Check sheet for the modelled part. Datum: model origin and axes. Units: mm. Face numbers are marked on the shaded views. A direction names the side the tool comes from. Round coordinates to 2 decimals unless told otherwise and drop trailing zeros. Write each loop counter-clockwise with the first axis right and the second up, starting at its lowest first coordinate (ties: lowest second). Pieces come first, ordered by that corner, then holes.
Item 1: Release check for a two-part mould opening along Y. For the marked faces 1, 2 and 3 record: +Y half, -Y half, draft (parallel to the pull), parting line (faces both ways), or undercut.
Item 2: Tool access check on the marked faces 4, 5 and 6. Record the directions out of +Z, -Z, +X, -X, +Y, -Y that give a thin tool (end or side, any length) a straight path to the whole face; none if there is none.
Item 3: Cross-section at C-C on z = -5. Enter the section's corners in (x, y), plus the area to 3 significant figures.
Item 4: Material ranges on line 1 (X direction, y = 3, z = -8.5); line 2 (Y direction, x = 3.25, z = -14.25); line 3 (Y direction, x = 6.5, z = -8.25), recorded low to high.
Item 5: Cross-section at B-B on y = 4.5. Enter the section's corners in (x, z), plus the area to 3 significant figures.
Item 6: Go/stop test with flat-tipped pins: pin 1 Ø1.5 at (y, z) = (5, -9) entering from -X; pin 2 Ø3.5 at (y, z) = (4.5, -6.5) entering from +X; pin 3 Ø2 at (x, y) = (9.5, 4.5) entering from -Z; pin 4 Ø1.5 at (x, z) = (9, -11.5) entering from -Y. Record where each tip stops, or that it passes through.
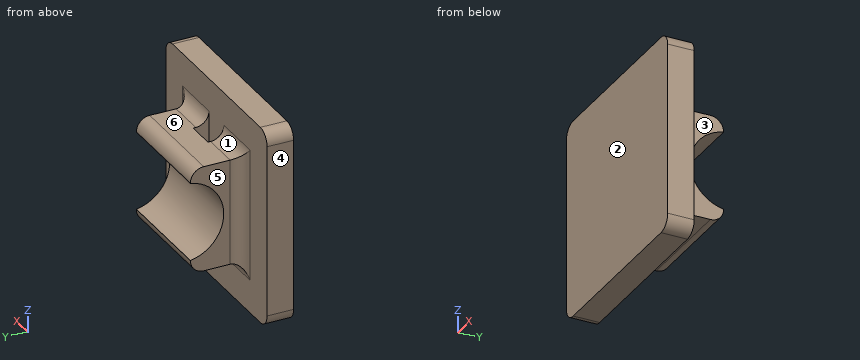
from build123d import *

# Parameters (mm, degrees)
CROQUIS1_W              = 15
CROQUIS1_H              = 15
SALIENTE_EXTRUIR1_DEPTH = 2
CROQUIS2_W              = 8
CROQUIS2_H              = 8
SALIENTE_EXTRUIR2_DEPTH = 4
CROQUIS3_R              = 3
CORTAR_EXTRUIR1_DEPTH   = 8
CROQUIS4_W              = 2.2
CROQUIS4_H              = 1.2
CORTAR_EXTRUIR3_DEPTH   = 8
REDONDEO1_R             = 1


with BuildPart() as part:
    # Croquis1 → Saliente-Extruir1 (new body)
    with BuildSketch(Plane(origin=(0, 0, 0), x_dir=(1, 0, 0), z_dir=(0, 1, 0))):
        with Locations((7.5, 7.5)):
            Rectangle(CROQUIS1_W, CROQUIS1_H)
    extrude(amount=SALIENTE_EXTRUIR1_DEPTH)

    # Croquis2 → Saliente-Extruir2 (add)
    with BuildSketch(Plane(origin=(0, 2, 0), x_dir=(1, 0, 0), z_dir=(0, 1, 0))):
        with Locations((7.5, 7.5)):
            Rectangle(CROQUIS2_W, CROQUIS2_H)
    extrude(amount=SALIENTE_EXTRUIR2_DEPTH)

    # Croquis3 → Cortar-Extruir1 (cut)
    with BuildSketch(Plane(origin=(11.5, 0, 0), x_dir=(0, 0, -1), z_dir=(1, 0, 0))):
        with Locations((7.5, 6.485438982)):
            Circle(CROQUIS3_R)
    extrude(amount=-CORTAR_EXTRUIR1_DEPTH, mode=Mode.SUBTRACT)

    # Croquis4 → Cortar-Extruir3 (cut)
    with BuildSketch(Plane.XY.offset(-3.5)):
        with Locations((7.5, 2.6)):
            Rectangle(CROQUIS4_W, CROQUIS4_H)
    extrude(amount=-CORTAR_EXTRUIR3_DEPTH, mode=Mode.SUBTRACT)

    # Redondeo1
    redondeo1_edges = [part.edges().sort_by_distance(p)[0] for p in [
        (11.5, 2, -7.5),
        (10.05, 2, -11.5),
        (3.5, 2, -7.5),
        (4.95, 2, -3.5),
        (7.5, 6, -11.5),
        (7.5, 6, -3.5),
        (10.05, 2, -3.5),
        (4.95, 2, -11.5),
        (0, 1, -15),
        (15, 1, -15),
        (15, 1, 0),
        (0, 1, 0),
    ]]
    fillet(redondeo1_edges, radius=REDONDEO1_R)


solid = part.part
Response values:
1. face 1: +Y half
1. face 2: -Y half
1. face 3: draft
2. face 4: +Z, -Z, -X, +Y, -Y
2. face 5: +Z, -Z, -X, +Y
2. face 6: +Z, +X, -X, +Y
3. outline: (0, 0) - (15, 0) - (15, 2) - (12.5, 2) arc R1 cw to (11.5, 3) - (11.5, 4.83) - (3.5, 4.83) - (3.5, 3) arc R1 cw to (2.5, 2) - (0, 2) - close; hole (6.4, 2) - (8.6, 2) - (8.6, 3.2) - (6.4, 3.2) - close
3. area: 50.4 mm2
4. line 1: x = 3.5 to 6.4, 8.6 to 11.5
4. line 2: y = 0 to 2
4. line 3: y = 0 to 2, 3.2 to 3.58
5. outline: (3.5, -11.5) - (11.5, -11.5) - (11.5, -9.75) - (3.5, -9.75) - close; (3.5, -5.25) - (11.5, -5.25) - (11.5, -3.5) - (3.5, -3.5) - close
5. area: 28.0 mm2
6. pin 1: passes through
6. pin 2: stops at x = 11.53
6. pin 3: stops at z = -11.5
6. pin 4: stops at y = 0
